```python
from build123d import *

# Parameters (mm, degrees)
SKETCH1_W                = 165
SKETCH1_H                = 225
BOSS_EXTRUDE1_DEPTH      = 8
SKETCH2_W                = 40
SKETCH2_H                = 70
CUT_EXTRUDE1_DEPTH       = 280.130793715
CHAMFER1_SIZE            = 60
M6_CLEARANCE_HOLE1_D     = 6.4
M6_CLEARANCE_HOLE1_DEPTH = 8
M6_CLEARANCE_HOLE1_TIP   = 1.922753981
M5_CLEARANCE_HOLE1_D     = 5.3
M5_CLEARANCE_HOLE1_DEPTH = 8
M5_CLEARANCE_HOLE1_TIP   = 1.59228064
M5_CLEARANCE_HOLE2_D     = 5.3
M5_CLEARANCE_HOLE2_DEPTH = 8
M5_CLEARANCE_HOLE2_TIP   = 1.59228064
FILLET1_R                = 3
M4_CLEARANCE_HOLE1_D     = 4.3
M4_CLEARANCE_HOLE1_DEPTH = 8
M4_CLEARANCE_HOLE1_TIP   = 1.291850331


with BuildPart() as part:
    # Sketch1 → Boss-Extrude1 (new body)
    with BuildSketch(Plane(origin=(0, 0, 0), x_dir=(1, 0, 0), z_dir=(0, 1, 0))):
        with Locations((82.5, 112.5)):
            Rectangle(SKETCH1_W, SKETCH1_H)
    extrude(amount=BOSS_EXTRUDE1_DEPTH)

    # Sketch2 → Cut-Extrude1 (cut, through all)
    with BuildSketch(Plane.XZ):
        with Locations((20, -82.5)):
            Rectangle(SKETCH2_W, SKETCH2_H)
    extrude(amount=-CUT_EXTRUDE1_DEPTH, mode=Mode.SUBTRACT)

    # Chamfer1
    chamfer1_edges = [part.edges().sort_by_distance(p)[0] for p in [
        (0, 4, -225),
        (165, 4, -225),
    ]]
    chamfer(chamfer1_edges, length=CHAMFER1_SIZE)

    # M6 Clearance Hole1
    with Locations(Plane(origin=(0, 8, 0), x_dir=(1, 0, 0), z_dir=(0, 1, 0))):
        with Locations((82.5, 210)):
            Hole(M6_CLEARANCE_HOLE1_D / 2, depth=M6_CLEARANCE_HOLE1_DEPTH)
            with Locations((0, 0, -(M6_CLEARANCE_HOLE1_DEPTH + M6_CLEARANCE_HOLE1_TIP / 2))):  # 118° drill point
                Cone(0, M6_CLEARANCE_HOLE1_D / 2, M6_CLEARANCE_HOLE1_TIP, mode=Mode.SUBTRACT)

    # M5 Clearance Hole1
    with Locations(Plane(origin=(0, 8, 0), x_dir=(1, 0, 0), z_dir=(0, 1, 0))):
        with Locations((7.5, 158.5), (37.5, 158.5), (37.5, 126.5), (7.5, 126.5), (157.5, 126.5), (127.5, 126.5), (127.5, 158.5), (157.5, 158.5), (157.5, 6.5), (127.5, 6.5), (127.5, 38.5), (157.5, 38.5), (7.5, 38.5), (37.5, 38.5), (37.5, 6.5), (7.5, 6.5)):
            Hole(M5_CLEARANCE_HOLE1_D / 2, depth=M5_CLEARANCE_HOLE1_DEPTH)
            with Locations((0, 0, -(M5_CLEARANCE_HOLE1_DEPTH + M5_CLEARANCE_HOLE1_TIP / 2))):  # 118° drill point
                Cone(0, M5_CLEARANCE_HOLE1_D / 2, M5_CLEARANCE_HOLE1_TIP, mode=Mode.SUBTRACT)

    # M5 Clearance Hole2
    with Locations(Plane(origin=(0, 8, 0), x_dir=(1, 0, 0), z_dir=(0, 1, 0))):
        with Locations((56.5, 26), (82.5, 26), (108.5, 26), (82.5, 52), (108.5, 52), (82.5, 78), (108.5, 78), (82.5, 104), (108.5, 104), (82.5, 130), (108.5, 130), (82.5, 156), (108.5, 156), (82.5, 182), (108.5, 182), (56.5, 52), (56.5, 78), (56.5, 104), (56.5, 130), (56.5, 156), (56.5, 182)):
            Hole(M5_CLEARANCE_HOLE2_D / 2, depth=M5_CLEARANCE_HOLE2_DEPTH)
            with Locations((0, 0, -(M5_CLEARANCE_HOLE2_DEPTH + M5_CLEARANCE_HOLE2_TIP / 2))):  # 118° drill point
                Cone(0, M5_CLEARANCE_HOLE2_D / 2, M5_CLEARANCE_HOLE2_TIP, mode=Mode.SUBTRACT)

    # Fillet1
    fillet1_edges = [part.edges().sort_by_distance(p)[0] for p in [
        (0, 4, -117.5),
        (0, 4, -47.5),
        (40, 4, -47.5),
        (40, 4, -117.5),
        (60, 4, -225),
        (105, 4, -225),
        (165, 4, -165),
        (0, 4, -165),
        (165, 4, 0),
        (0, 4, 0),
    ]]
    fillet(fillet1_edges, radius=FILLET1_R)

    # M4 Clearance Hole1
    with Locations(Plane(origin=(0, 8, 0), x_dir=(1, 0, 0), z_dir=(0, 1, 0))):
        with Locations((144, 105.5), (159, 105.5), (159, 59.5), (144, 59.5)):
            Hole(M4_CLEARANCE_HOLE1_D / 2, depth=M4_CLEARANCE_HOLE1_DEPTH)
            with Locations((0, 0, -(M4_CLEARANCE_HOLE1_DEPTH + M4_CLEARANCE_HOLE1_TIP / 2))):  # 118° drill point
                Cone(0, M4_CLEARANCE_HOLE1_D / 2, M4_CLEARANCE_HOLE1_TIP, mode=Mode.SUBTRACT)


solid = part.part
```
Part model, mm, in its own coordinate system. A direction names the side the tool comes from. Round coordinates to 2 decimals unless told otherwise and drop trailing zeros. Order: outer loops, then holes, each group sorted by start corner. A loop starts at its lowest first (then second) coordinate and runs counter-clockwise, first axis right, second up. Notation, with made-up numbers: M 48.5,42 L 99.5,42 A34 ccw 99.5,80 Z; hole C 71.5,44.5 d4. An arc over 180 degrees is marked long. Put each result on its own line as item: value. Start each with the question number.
1. Slice it at A-A on x = 21. List the corners of the cut face in (y, z), then the cut area to 3 significant figures.
2. Two-plate mould, pull along Z, no slides. Class faces 3 (the face through (0, 4, -142)), 4 (the face through (39.453, 3.944, -160.291)): +Z half, -Z half, draft (parallel to the pull), parting line (faces both ways), or undercut.
3. Drill centre lines: probe 1 along X at (y, z) = (2, -38.5); probe 2 along X at (y, z) = (3.25, -130); probe 3 along X at (y, z) = (3.5, -78). Where is each one in solid material? Low to high. Write a range as [from, to].
4. Slice it at B-B on x = 108.5. State how many separate pieces and enclosed holes the cut face has, then the cut area to 3 significant figures.
5. Tool access for faces 1 (the face through (53.972, 3.944, -156.796)), 2 (the face through (40, 4, -83)): list every direction of +Z, -Z, +X, -X, +Y, -Y with a clear straight run to the whole face (end or side of a thin tool).
6. Slice it at C-C on x = 127.5. List the corners of the cut face in (y, z).
7. Drop flat-ended pins along their axis: pin 1 (8 mm diameter, centred on x = 80, z = -164, fed in from -Y); pin 2 (1 mm diameter, centred on y = 2.5, z = -61.5, fed in from -X); pin 3 (5 mm diameter, centred on x = 127.5, z = -158.5, fed in from +Y); pin 4 (4 mm diameter, centred on x = 27.5, y = 4.5, fed in from -Z). Give the stop position or say it passes through.
Findings:
1. outline: M 0,-186 L 8,-186 L 8,-117.5 L 0,-117.5 Z; M 0,-47.5 L 8,-47.5 L 8,0 L 0,0 Z
1. area: 928 mm2
2. face 3: draft
2. face 4: undercut
3. probe 1: [0, 4.85], [10.15, 34.85], [40.15, 124.85], [130.15, 154.85], [160.15, 165]
3. probe 2: [0, 53.85], [59.15, 79.85], [85.15, 105.85], [111.15, 165]
3. probe 3: [40, 53.85], [59.15, 79.85], [85.15, 105.85], [111.15, 165]
4. separate pieces: 8
4. enclosed holes: 0
4. area: 1,480 mm2
5. face 1: +Y, -Y
5. face 2: -X, +Y, -Y
6. outline: M 0,-202.5 L 8,-202.5 L 8,-161.15 L 0,-161.15 Z; M 0,-155.85 L 8,-155.85 L 8,-129.15 L 0,-129.15 Z; M 0,-123.85 L 8,-123.85 L 8,-41.15 L 0,-41.15 Z; M 0,-35.85 L 8,-35.85 L 8,-9.15 L 0,-9.15 Z; M 0,-3.85 L 8,-3.85 L 8,0 L 0,0 Z
7. pin 1: y = 0
7. pin 2: x = 40
7. pin 3: through
7. pin 4: z = -194.5
